Input: part model. Units: mm. Frame: model coordinates. A direction names the side the tool comes from. Give positions to 0.01 mm unless a question says otherwise; leave off trailing zeros. Write each loop counter-clockwise with the first axis right and the second up, starting at its lowest first coordinate (ties: lowest second). Pieces come first, ordered by that corner, then holes. Notation, with made-up numbers: (17.5, 74) -> (28.5, 74) arc R14 cw to (28.5, 86) -> close; hole circle Ø10 at (33.5, 28.5). An arc over 180 degrees is marked (long way). Answer as a JSON object with one key per item and string values. Group by question number.
Autodesk Inventor part; units mm, degrees
ref_plane "YZ Plane" through (0, 0, 0) normal (1, 0, 0) x (0, 1, 0)
ref_plane "XZ Plane" through (0, 0, 0) normal (0, 1, 0) x (-1, 0, 0)
ref_plane "XY Plane" through (0, 0, 0) normal (0, 0, 1) x (1, 0, 0)
sketch "Sketch1" plane through (0, 0, 0) normal (0, 0, 1) x (1, 0, 0)
  line L0 (-400, -1080) -> (400, -1080)
  line L1 (400, -1080) -> (400, 1080)
  line L2 (400, 1080) -> (-400, 1080)
  line L3 (-400, 1080) -> (-400, -1080)
  line L4 (-400, -1080) -> (400, 1080) construction
  line L5 (400, -1080) -> (-400, 1080) construction
  point P0 (0, 0)
  dimension "d0" = 800
  dimension "d1" = 2160
extrude "Plate1" add sketch "Sketch1" along normal blind 10
sketch "Sketch2" plane through (0, 0, 10) normal (0, 0, 1) x (1, 0, 0)
  line L0 (400, -1080) -> (-400, -1080)
  line L1 (400, 1080) -> (400, -1080)
  line L2 (-400, 1080) -> (400, 1080)
  line L3 (-400, -1080) -> (-400, 1080)
  circle A0 centre (0, -929.5) radius 35
  point P0 (0, 0)
  point P1 (0, -1080)
  dimension "d3" = 70
  dimension "d4" = 150.5
extrude "Extrusion1" cut sketch "Sketch2" against normal through all contours A0
pattern_linear "Rectangular Pattern1" count 9 spacing 250 along (0, 1, 0) of "Extrusion1"
sketch "Sketch3" plane through (0, 0, 0) normal (0, 0, -1) x (-1, 0, 0)
  line L0 (240, -1080) -> (180, -1080)
  line L1 (180, -1080) -> (180, 1080)
  line L2 (180, 1080) -> (240, 1080)
  line L3 (240, 1080) -> (240, -1080)
  line L4 (-180, -1080) -> (-240, -1080)
  line L5 (-240, -1080) -> (-240, 1080)
  line L6 (-240, 1080) -> (-180, 1080)
  line L7 (-180, 1080) -> (-180, -1080)
  line L8 (0, -1080) -> (0, 1305.1217) construction
  line L9 (400, -1080) -> (-400, -1080)
  line L10 (-400, 1080) -> (400, 1080)
  point P0 (0, 0)
  dimension "d10" = 60
  dimension "d11" = 360
extrude "Extrusion2" add sketch "Sketch3" along normal blind 60 contours L0 L1 L2 L3 | L4 L5 L6 L7
sketch "Sketch4" plane through (-400, 1080, 10) normal (0, 1, 0) x (1, 0, 0)
  line L0 (160, 70) -> (220, 70)
  line L1 (160, 70) -> (220, 70)
  line L2 (220, 70) -> (220, 130)
  line L3 (220, 130) -> (160, 130)
  line L4 (160, 130) -> (160, 70)
  line L5 (163, 127) -> (217, 127)
  line L6 (217, 127) -> (217, 73)
  line L7 (217, 73) -> (163, 73)
  line L8 (163, 73) -> (163, 127)
  point P0 (400, 10)
  dimension "d15" = 60
  dimension "d16" = 3
extrude "Extrusion3" add sketch "Sketch4" against normal up to surface (2160 mm away)
mirror "Mirror1" about plane through (0, 0, 0) normal (1, 0, 0) of "Extrusion3"
equation "\"d2\" = Thickness"
equation "\"BendReliefDepth\" = 0.5 * Thickness"
properties part number "ДМФ 067 крышка v2.0"
1. Line query: line 1 (X direction, y = -499.5, z = -106); line 2 (X direction, y = -179, z = 2); line 3 (X direction, y = 931, z = -60.5). Output: solid intervals per line, ascending.
2. Contact query for flat-ended pins moving along their axis: pin 1 Ø6 at (y, z) = (5, -69.5) entering from +X; pin 2 Ø1 at (x, y) = (-140, 8) entering from -Z; pin 3 Ø10 at (y, z) = (738, -75) entering from -X. Output: stop coordinate, or through.
3. Section A-A (y = -179.5). Return the cut outline in (x, z), plus the area to 3 significant figures.
4. Section D-D (x = 87.5). Return the cut outline in (y, z), plus the area to 3 significant figures.
5. Mould query, pull axis X, two halves, no side actions, for faces 1 (the face through (240, 15, -59)), 2 (the face through (-218, 1080, -17)), 3 (the face through (-0.9, 1035.51, 5.07)). Classes: pulls with the +X half, pulls with the -X half, needs draft (parallel to the pull), parting line crosses it, or undercut.
6. Section B-B (z = -38.5). Return the cut outline in (x, y).
7. Section C-C (y = 413.5). Return the cut outline in (x, z).
8. Reachability of faces 4 (the face through (319, 15, 0)), 5 (the face through (-180, 15, -59)), 6 (the face through (-183, 15, -90)) from +Z, -Z, +X, -X, +Y, -Y: full face, straight path, thin tool, end or side. Return the list, or none.
Working result:
{
 "1": {"line 1": "x = -240 to -237, -183 to -180, 180 to 183, 237 to 240", "line 2": "x = -400 to -35, 35 to 400", "line 3": "x = -240 to -180, 180 to 240"},
 "2": {"pin 1": "stops at x = 240", "pin 2": "stops at z = 0", "pin 3": "stops at x = -240"},
 "3": {"outline": "(-400, 0) -> (-240, 0) -> (-240, -120) -> (-180, -120) -> (-180, 0) -> (-35, 0) -> (-35, 10) -> (-400, 10) -> close; (35, 0) -> (180, 0) -> (180, -120) -> (240, -120) -> (240, 0) -> (400, 0) -> (400, 10) -> (35, 10) -> close; hole (-237, -117) -> (-183, -117) -> (-183, -63) -> (-237, -63) -> close; hole (183, -117) -> (237, -117) -> (237, -63) -> (183, -63) -> close", "area": "15,900 mm^2"},
 "4": {"outline": "(-1080, 0) -> (1080, 0) -> (1080, 10) -> (-1080, 10) -> close", "area": "21,600 mm^2"},
 "5": {"face 1": "pulls with the +X half", "face 2": "needs draft", "face 3": "undercut"},
 "6": {"outline": "(-240, -1080) -> (-180, -1080) -> (-180, 1080) -> (-240, 1080) -> close; (180, -1080) -> (240, -1080) -> (240, 1080) -> (180, 1080) -> close"},
 "7": {"outline": "(-400, 0) -> (-240, 0) -> (-240, -120) -> (-180, -120) -> (-180, 0) -> (180, 0) -> (180, -120) -> (240, -120) -> (240, 0) -> (400, 0) -> (400, 10) -> (-400, 10) -> close; hole (-237, -117) -> (-183, -117) -> (-183, -63) -> (-237, -63) -> close; hole (183, -117) -> (237, -117) -> (237, -63) -> (183, -63) -> close"},
 "8": {"face 4": "-Z, +X, +Y, -Y", "face 5": "-Z, +Y, -Y", "face 6": "+Y, -Y"}
}
